Input: part model. Units: mm. Frame: model coordinates. Face numbers are marked on the shaded views. Give positions to 0.01 mm unless a question says otherwise; leave off trailing zeros. Order: outer loops, then holes, each group sorted by start corner. A loop starts at its lowest first (then second) coordinate and runs counter-clockwise, first axis right, second up. Notation, with made-up numbers: (60.5, 50.25) - (108.5, 50.25) arc R13 cw to (108.5, 70.25) - close; hole circle Ø1 at (77, 53). An arc over 180 degrees is marked (long way). Answer in a Markdown table with one row per item. Add a question column.
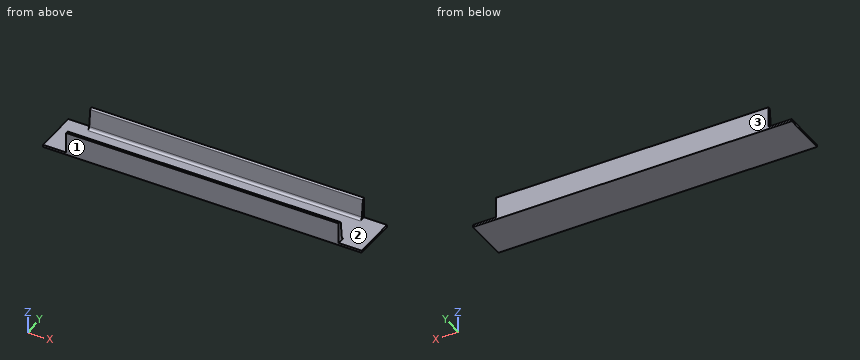
from build123d import *

# Parameters (mm, degrees)
C_CHANNEL_120_X_12_1_DEPTH = 900
CUT_EXTRUDE1_DEPTH         = 65


with BuildPart() as part:
    # Sketch12 → C channel 120 X 12(1) (new body)
    with BuildSketch(Plane.ZY):
        with BuildLine():
            Line((65, 125), (0, 125))
            Line((0, 125), (0, 0))
            Line((0, 0), (65, 0))
            Line((65, 0), (65, 5.845330836))
            ThreePointArc((65, 5.845330836), (63.844151715, 8.856418565), (60.970378085, 10.320679365))
            Line((60.970378085, 10.320679365), (13.463772294, 15.313824837))
            ThreePointArc((13.463772294, 15.313824837), (8.354841396, 17.916955149), (6.3, 23.27))
            Line((6.3, 23.27), (6.3, 106.74))
            ThreePointArc((6.3, 106.74), (8.354841396, 112.093044851), (13.463772294, 114.696175163))
            Line((13.463772294, 114.696175163), (60.970378085, 119.689320635))
            ThreePointArc((60.970378085, 119.689320635), (63.844151715, 121.153581435), (65, 124.164669164))
            Line((65, 124.164669164), (65, 125))
        make_face()
    extrude(amount=C_CHANNEL_120_X_12_1_DEPTH)

    # Sketch13 → Cut-Extrude1 (cut)
    with BuildSketch(Plane(origin=(0, 0, 0), x_dir=(0, 0, -1), z_dir=(1, 0, 0))):
        Polygon((-6.3, 106.74), (-6.3, 128.866505143), (-71.707289192, 128.866505143), (-71.707289192, -13.872532072), (-6.3, -13.872532072), align=None)
    cut_extrude1 = extrude(amount=-CUT_EXTRUDE1_DEPTH, mode=Mode.SUBTRACT)

    # Mirror1: Cut-Extrude1 across plane
    add(cut_extrude1.mirror(Plane(origin=(-450, 0, 0), x_dir=(0, 0, 1), z_dir=(1, 0, 0))), mode=Mode.SUBTRACT)


solid = part.part
Q1. Section B-B, the plane x = -552. Return loops of the section in (y, z), then the cut area to 3 significant figures.
Q2. Contact query for flat-ended pins moving along their axis: P1, Ø5.5, axis at y = 117, z = 32, coming from the +X side; P2, Ø11.5, axis at y = 14.5, z = 38, coming from the -X side. Output: stop coordinate, or through.
Q3. Pull-direction query (Y, two-part tool) for the marked faces 1, 2 and 3; classes: +Y half, -Y half, draft (parallel to the pull), parting line (faces both ways), or undercut.
Q4. Line query: probe 1 along Y at (x, z) = (-127.5, 60); probe 2 along Y at (x, z) = (-758, 12.5); probe 3 along Z at (x, y) = (-449.5, 70.5). Output: solid intervals per line, ascending.
Q5. Section C-C, the plane y = 70.5. Return loops of the section in (x, z), then the cut area to 3 significant figures.
Q6. Section A-A, the plane z = 43. Return loops of the section in (x, y), then the cut area to 3 significant figures.
Computed:
| question | item | result |
|---|---|---|
| 1 | outline | (0, 0) - (125, 0) - (125, 65) - (124.16, 65) arc R4.5 ccw to (119.69, 60.97) - (114.7, 13.46) arc R8 cw to (106.74, 6.3) - (23.27, 6.3) arc R8 cw to (15.31, 13.46) - (10.32, 60.97) arc R4.5 ccw to (5.85, 65) - (0, 65) - close |
| 1 | area | 2,030 mm^2 |
| 2 | P1 | stops at x = -65 |
| 2 | P2 | stops at x = -835 |
| 3 | face 1 | -Y half |
| 3 | face 2 | undercut |
| 3 | face 3 | +Y half |
| 4 | probe 1 | y = 0 to 10.42, 119.59 to 125 |
| 4 | probe 2 | y = 0 to 15.48, 114.53 to 125 |
| 4 | probe 3 | z = 0 to 6.3 |
| 5 | outline | (-900, 0) - (0, 0) - (0, 6.3) - (-900, 6.3) - close |
| 5 | area | 5,670 mm^2 |
| 6 | outline | (-835, 0) - (-65, 0) - (-65, 12.21) - (-835, 12.21) - close; (-835, 117.8) - (-65, 117.8) - (-65, 125) - (-835, 125) - close |
| 6 | area | 14,900 mm^2 |
